Build history of the part. All positions in model axes, mm. Give positions to 0.01 mm unless a question says otherwise; leave off trailing zeros. Write each loop counter-clockwise with the first axis right and the second up, starting at its lowest first coordinate (ties: lowest second). Pieces come first, ordered by that corner, then holes. Notation, with made-up numbers: (-14, 43.5) -> (10, 43.5) arc R36 ccw to (10, 78.5) -> close; hole circle Ø3 at (-1, 57.25). An arc over 180 degrees is marked (long way). Put each result on its own line as item: value. Start each with the question number.
Item 1: Slice it at C-C, the plane z = 0.85. Give the number of separate pieces and of enclosed holes in the cut face, plus the area to 3 significant figures.
Item 2: Flat gauge pins, fed straight in: pin 1 Ø6 at (x, y) = (95, 57.5) entering from +Z; pin 2 Ø5 at (x, y) = (42, 38.5) entering from -Z. Where does each tip first touch, or does it go through?
Item 3: Drill centre lines: line 1 along X through (y, z) = (36, 1.35); line 2 along Y through (x, z) = (19, 0.95); line 3 along Y through (x, z) = (52, 1.3). Where is each one in solid material? Low to high.
Item 4: Slice it at A-A, the plane y = 90. List the corners of the cut face in (x, z), plus the area to 3 significant figures.
Item 5: Slice it at B-B, the plane x = 149.5. List the corners of the cut face in (y, z), plus the area to 3 significant figures.
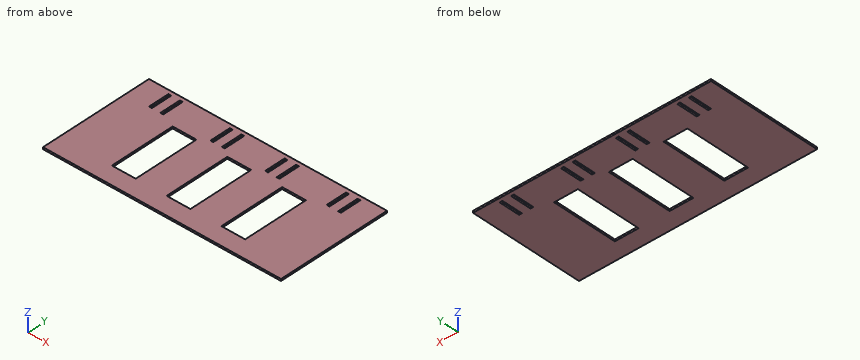
```python
from build123d import *

# Parameters (mm, degrees)
SKETCH_1_W          = 250
SKETCH_1_H          = 120
EXTRUDE_1_DEPTH     = 2
SKETCH_2_W          = 3
SKETCH_2_H          = 22
CUT_EXTRUDE_1_DEPTH = 2
SKETCH_4_W          = 25
SKETCH_4_H          = 68.757414634
CUT_EXTRUDE_3_DEPTH = 10


with BuildPart() as part:
    # 草图1 → 凸台-拉伸1 (new body)
    with BuildSketch(Plane.XY):
        with Locations((85.581519181, 72.657914473)):
            Rectangle(SKETCH_1_W, SKETCH_1_H)
    extrude(amount=EXTRUDE_1_DEPTH)

    # 草图2 → 切除-拉伸1 (cut)
    with BuildSketch(Plane.XY.offset(2)):
        with Locations((-13.718480819, 117.592867426)):
            Rectangle(SKETCH_2_W, SKETCH_2_H)
        with Locations((-1.718480819, 117.592867426)):
            Rectangle(SKETCH_2_W, SKETCH_2_H)
        with Locations((50.831519181, 117.592867426)):
            Rectangle(SKETCH_2_W, SKETCH_2_H)
        with Locations((62.831519181, 117.592867426)):
            Rectangle(SKETCH_2_W, SKETCH_2_H)
        with Locations((108.331519181, 117.592867426)):
            Rectangle(SKETCH_2_W, SKETCH_2_H)
        with Locations((120.331519181, 117.592867426)):
            Rectangle(SKETCH_2_W, SKETCH_2_H)
        with Locations((172.881519181, 117.592867426)):
            Rectangle(SKETCH_2_W, SKETCH_2_H)
        with Locations((184.881519181, 117.592867426)):
            Rectangle(SKETCH_2_W, SKETCH_2_H)
    extrude(amount=-CUT_EXTRUDE_1_DEPTH, mode=Mode.SUBTRACT)

    # 草图4 → 切除-拉伸3 (cut)
    with BuildSketch(Plane(origin=(0, 0, 0), x_dir=(-1, 0, 0), z_dir=(0, 0, -1))):
        with Locations((-143.081519181, 65.748927638)):
            Rectangle(SKETCH_4_W, SKETCH_4_H)
        with Locations((-85.581519181, 65.748927638)):
            Rectangle(SKETCH_4_W, SKETCH_4_H)
        with Locations((-28.081519181, 65.748927638)):
            Rectangle(SKETCH_4_W, SKETCH_4_H)
    extrude(amount=-CUT_EXTRUDE_3_DEPTH, mode=Mode.SUBTRACT)


solid = part.part
```
Values follow:
1. separate pieces: 1
1. enclosed holes: 11
1. area: 24,300 mm2
2. pin 1: through
2. pin 2: z = 0
3. line 1: -39.42 to 15.58, 40.58 to 73.08, 98.08 to 130.58, 155.58 to 210.58
3. line 2: 12.66 to 31.37, 100.13 to 132.66
3. line 3: 12.66 to 106.59, 128.59 to 132.66
4. outline: (-39.42, 0) -> (15.58, 0) -> (15.58, 2) -> (-39.42, 2) -> close; (40.58, 0) -> (73.08, 0) -> (73.08, 2) -> (40.58, 2) -> close; (98.08, 0) -> (130.58, 0) -> (130.58, 2) -> (98.08, 2) -> close; (155.58, 0) -> (210.58, 0) -> (210.58, 2) -> (155.58, 2) -> close
4. area: 350 mm2
5. outline: (12.66, 0) -> (31.37, 0) -> (31.37, 2) -> (12.66, 2) -> close; (100.13, 0) -> (132.66, 0) -> (132.66, 2) -> (100.13, 2) -> close
5. area: 102 mm2
